Design review of the part built by this model. Coordinates are the model's own, in mm. A direction names the side the tool comes from. Give positions to 0.01 mm unless a question says otherwise; leave off trailing zeros. Loops run counter-clockwise (first coordinate to the right, second up) from the corner with the lowest first, then second, coordinate; pieces in that order, holes last. Notation, with made-up numbers: M -16.5,-21 L -12.5,-21 A25 ccw -12.5,10 Z; hole C -19,78 d5. An arc over 180 degrees is marked long. Answer as CSV lines item,"result".
```python
from build123d import *

# Parameters (mm, degrees)
SKETCH1_W               = 276.86
SKETCH1_H               = 163.5252
SKETCH1_W_2             = 260.9596
SKETCH1_H_2             = 138.1252
BOSS_EXTRUDE1_DEPTH     = 31.75
SKETCH2_R               = 4.953
CUT_EXTRUDE1_DEPTH      = 291.421495173
SKETCH3_R               = 1.27
BOSS_EXTRUDE2_DEPTH     = 31.75
MIRROR4_COPY_1_SKETCH_R = 1.27
MIRROR4_COPY_1_DEPTH    = 31.75
FILLET2_R               = 1.524
SKETCH4_W               = 25.781
SKETCH4_H               = 13.081
CUT_EXTRUDE2_DEPTH      = 3.175
CUT_EXTRUDE3_REACH      = 223.668
SKETCH5_R               = 1.27
CUT_EXTRUDE4_DEPTH      = 170.004206297
SKETCH7_R               = 3.556
BOSS_EXTRUDE3_DEPTH     = 4.7752
FILLET3_R               = 9.525


with BuildPart() as part:
    # Sketch1 → Boss-Extrude1 (new body)
    with BuildSketch(Plane(origin=(0, 0, 0), x_dir=(1, 0, 0), z_dir=(0, 1, 0))):
        Rectangle(SKETCH1_W, SKETCH1_H)
        Rectangle(SKETCH1_W_2, SKETCH1_H_2, mode=Mode.SUBTRACT)
    extrude(amount=BOSS_EXTRUDE1_DEPTH)

    # Sketch2 → Cut-Extrude1 (cut, through all)
    with BuildSketch(Plane(origin=(138.43, 0, 0), x_dir=(0, 0, -1), z_dir=(1, 0, 0))):
        with Locations((0, 31.75)):
            Circle(SKETCH2_R)
        with Locations((43.1038, 31.75)):
            Circle(SKETCH2_R)
        with Locations((-43.1038, 31.75)):
            Circle(SKETCH2_R)
    extrude(amount=-CUT_EXTRUDE1_DEPTH, mode=Mode.SUBTRACT)

    # Sketch3 → Boss-Extrude2 (add, through all)
    with BuildSketch(Plane(origin=(0, 31.75, 0), x_dir=(1, 0, 0), z_dir=(0, 1, 0))):
        with BuildLine():
            Line((-138.43, 81.7626), (-138.43, 86.8426))
            ThreePointArc((-138.43, 86.8426), (-133.6675, 91.6051), (-128.905, 86.8426))
            Line((-128.905, 86.8426), (-128.905, 81.7626))
            Line((-128.905, 81.7626), (-138.43, 81.7626))
        make_face()
        with Locations(Location((-133.6675, 86.8426, 0), (0, 0, 270))):
            Circle(SKETCH3_R, mode=Mode.SUBTRACT)
    boss_extrude2 = extrude(amount=-BOSS_EXTRUDE2_DEPTH)

    # Mirror3: Boss-Extrude2 across plane
    add(boss_extrude2.mirror(Plane(origin=(0, 0, 0), x_dir=(0, 0, 1), z_dir=(1, 0, 0))))

    # Mirror4: Boss-Extrude2 across plane
    add(boss_extrude2.mirror(Plane.XY))

    # Mirror4 copy 1 sketch → Mirror4 copy 1 (add, through all)
    with BuildSketch(Plane(origin=(0, 31.75, 0), x_dir=(-1, 0, 0), z_dir=(0, 1, 0))):
        with BuildLine():
            Line((-138.43, 81.7626), (-138.43, 86.8426))
            ThreePointArc((-138.43, 86.8426), (-133.6675, 91.6051), (-128.905, 86.8426))
            Line((-128.905, 86.8426), (-128.905, 81.7626))
            Line((-128.905, 81.7626), (-138.43, 81.7626))
        make_face()
        with Locations(Location((-133.6675, 86.8426, 0), (0, 0, 270))):
            Circle(MIRROR4_COPY_1_SKETCH_R, mode=Mode.SUBTRACT)
    extrude(amount=-MIRROR4_COPY_1_DEPTH)

    # Fillet2
    fillet2_edges = [part.edges().sort_by_distance(p)[0] for p in [
        (-128.905, 15.875, 81.7626),
        (128.905, 15.875, 81.7626),
        (-128.905, 15.875, -81.7626),
        (128.905, 15.875, -81.7626),
    ]]
    fillet(fillet2_edges, radius=FILLET2_R)

    # Sketch4 → Cut-Extrude2 (cut)
    with BuildSketch(Plane(origin=(0, 0, -81.7626), x_dir=(-1, 0, 0), z_dir=(0, 0, -1))):
        with Locations((0, 31.75)):
            Rectangle(SKETCH4_W, SKETCH4_H)
    cut_extrude2 = extrude(amount=-CUT_EXTRUDE2_DEPTH, mode=Mode.SUBTRACT)

    # Sketch5 → Cut-Extrude3 (cut, up to next)
    with BuildSketch(Plane(origin=(0, 0, -78.5876), x_dir=(-1, 0, 0), z_dir=(0, 0, -1)), mode=Mode.PRIVATE) as cut_extrude3_sk1:
        with Locations((-6.35, 28.575)):
            Circle(SKETCH5_R)
    cut_extrude3_tool1 = extrude(cut_extrude3_sk1.sketch, amount=-CUT_EXTRUDE3_REACH, mode=Mode.PRIVATE) & part.part
    # Sketch5 → Cut-Extrude3 (cut, up to next)
    with BuildSketch(Plane(origin=(0, 0, -78.5876), x_dir=(-1, 0, 0), z_dir=(0, 0, -1)), mode=Mode.PRIVATE) as cut_extrude3_sk2:
        with Locations((6.35, 28.575)):
            Circle(SKETCH5_R)
    cut_extrude3_tool2 = extrude(cut_extrude3_sk2.sketch, amount=-CUT_EXTRUDE3_REACH, mode=Mode.PRIVATE) & part.part
    cut_extrude3_1 = cut_extrude3_tool1.solids().sort_by_distance((6.35, 28.575, -78.5876))[0]
    add(cut_extrude3_1, mode=Mode.SUBTRACT)
    cut_extrude3_2 = cut_extrude3_tool2.solids().sort_by_distance((-6.35, 28.575, -78.5876))[0]
    add(cut_extrude3_2, mode=Mode.SUBTRACT)
    cut_extrude3 = cut_extrude3_1 + cut_extrude3_2  # Cut-Extrude3 as one shape, for the pattern or mirror that repeats it

    # Mirror5: Cut-Extrude2, Cut-Extrude3 across plane
    add(cut_extrude2.mirror(Plane.XY), mode=Mode.SUBTRACT)
    add(cut_extrude3.mirror(Plane.XY), mode=Mode.SUBTRACT)

    # Sketch6 → Cut-Extrude4 (cut, through all)
    with BuildSketch(Plane(origin=(0, 31.75, 0), x_dir=(1, 0, 0), z_dir=(0, 1, 0))):
        Polygon((0, 0), (0, 94.782822777), (154.500251477, 94.782822777), (154.500251477, -104.416951251), (0, -98.891495214), align=None)
    extrude(amount=-CUT_EXTRUDE4_DEPTH, mode=Mode.SUBTRACT)

    # Sketch7 → Boss-Extrude3 (add)
    with BuildSketch(Plane.XZ):
        with BuildLine():
            Line((-138.43, 81.7626), (-147.955, 81.7626))
            ThreePointArc((-147.955, 81.7626), (-157.48, 72.2376), (-147.955, 62.7126))
            Line((-147.955, 62.7126), (-138.43, 62.7126))
            Line((-138.43, 62.7126), (-138.43, 81.7626))
        make_face()
        with Locations(Location((-147.955, 72.2376, 0), (0, 0, 270))):
            Circle(SKETCH7_R, mode=Mode.SUBTRACT)
    boss_extrude3 = extrude(amount=-BOSS_EXTRUDE3_DEPTH)

    # Mirror6: Boss-Extrude3 across plane
    add(boss_extrude3.mirror(Plane.XY))

    # Fillet3
    fillet3_edges = [part.edges().sort_by_distance(p)[0] for p in [
        (-138.43, 2.3876, -62.7126),
        (-138.43, 2.3876, 62.7126),
    ]]
    fillet(fillet3_edges, radius=FILLET3_R - 0.0001)  # a hair under: the kernel refuses the full size


solid = part.part
```
1. We need section A-A, the plane x = -104. Write out the cut boundary in (y, z), plus the area to 3 significant figures.
Answer block:
outline,"M 0,-81.76 L 31.75,-81.76 L 31.75,-69.06 L 0,-69.06 Z; M 0,69.06 L 31.75,69.06 L 31.75,81.76 L 0,81.76 Z"
area,"806 mm²"
2. For faces 4 (the cylindrical face through (-141.1, 2.4, 59.8)), 5 (the flat face through (-8, 29, 78.588)), 6 (the flat face through (-66, 16, 69.063)), list the 3-axis set-ups (+Z, -Z, +X, -X, +Y, -Y) from which the entire face can be reached by the end or side of a thin tool; tool diameter is ignored.
Answer block:
face 4,"-X, +Y, -Y"
face 5,"+Z, +X, +Y"
face 6,"+X, +Y, -Y"
3. The part is to be moulded in two halves that separate along X. For faces 1 (the cylindrical face through (-133.772, 16.097, 91.604)), 2 (the cylindrical face through (-151.426, 2.354, 73.008)), 3 (the flat face through (-135, 31.75, -22)), say which applies: pulls with the +X half, pulls with the -X half, needs draft (parallel to the pull), parting line crosses it, or undercut.
Answer block:
face 1,"parting line crosses it"
face 2,"undercut"
face 3,"needs draft"
4. We need section D-D, the plane z = 66.5. Write out the cut boundary in (x, y).
Answer block:
outline,"M -155.56,0 L -130.48,0 L -130.48,31.75 L -138.43,31.75 L -138.43,4.78 L -155.56,4.78 Z"
5. We need section B-B, the plane y = 18. Write out the cut boundary in (x, z) (1 decimal), plus the area to 3 significant figures.
Answer block:
outline,"M -138.4,-86.8 A4.8 ccw -128.9,-86.8 L -128.9,-83.3 A1.5 cw -127.4,-81.8 L 0,-81.8 L 0,-69.1 L -130.5,-69.1 L -130.5,69.1 L 0,69.1 L 0,81.8 L -127.4,81.8 A1.5 cw -128.9,83.3 L -128.9,86.8 A4.8 ccw -138.4,86.8 Z; hole C -133.7,-86.8 d2.5; hole C -133.7,86.8 d2.5"
area,"4,770 mm²"
6. We need section C-C, the plane z = 16.5. Write out the cut boundary in (x, y).
Answer block:
outline,"M -138.43,0 L -130.48,0 L -130.48,31.75 L -138.43,31.75 Z"
7. To check wall thickness, follow L1, parallel to Z at x = -14, y = 9.5; L2, parallel to Z at x = -7.5, y = 29.5; L3, parallel to Y at x = -6.35, z = -75 (3 decimals). State the ranges of each line that lie inside material, in increasing order. Write a range as [from, to].
Answer block:
L1,"[-81.76, -69.06], [69.06, 81.76]"
L2,"[-78.59, -69.06], [69.06, 78.59]"
L3,"[0, 27.305], [29.845, 31.75]"
8. For P1, Ø12, axis at x = -127.5, y = 10.5, coming from the -Z side; P2, Ø6, axis at x = -81.5, y = 4, coming from the +Z side; P3, Ø9.5, axis at y = 16, z = -26.5, coming from the -X side, all flat-tipped, find the tip position at first contact; note any pin that passes through.
Answer block:
P1,"z = -91.6"
P2,"z = 81.76"
P3,"x = -138.43"
